Geometry: see drawing. Coordinates: mm, zero at the bounding-box minimum. Give positions to 0.01 mm unless a question says otherwise; leave off trailing zeros. Order: outer loops, then holes, each group sorted by start corner. A loop starts at its lowest first (then second) coordinate and runs counter-clockwise, first axis right, second up. Notation, with made-up numbers: M 3.5,43.25 L 57.5,43.25 A23 ccw 57.5,79.25 Z; hole C 82.5,-27.5 d5. An arc over 180 degrees is marked long. Return JSON: item names as keys, results as strings.
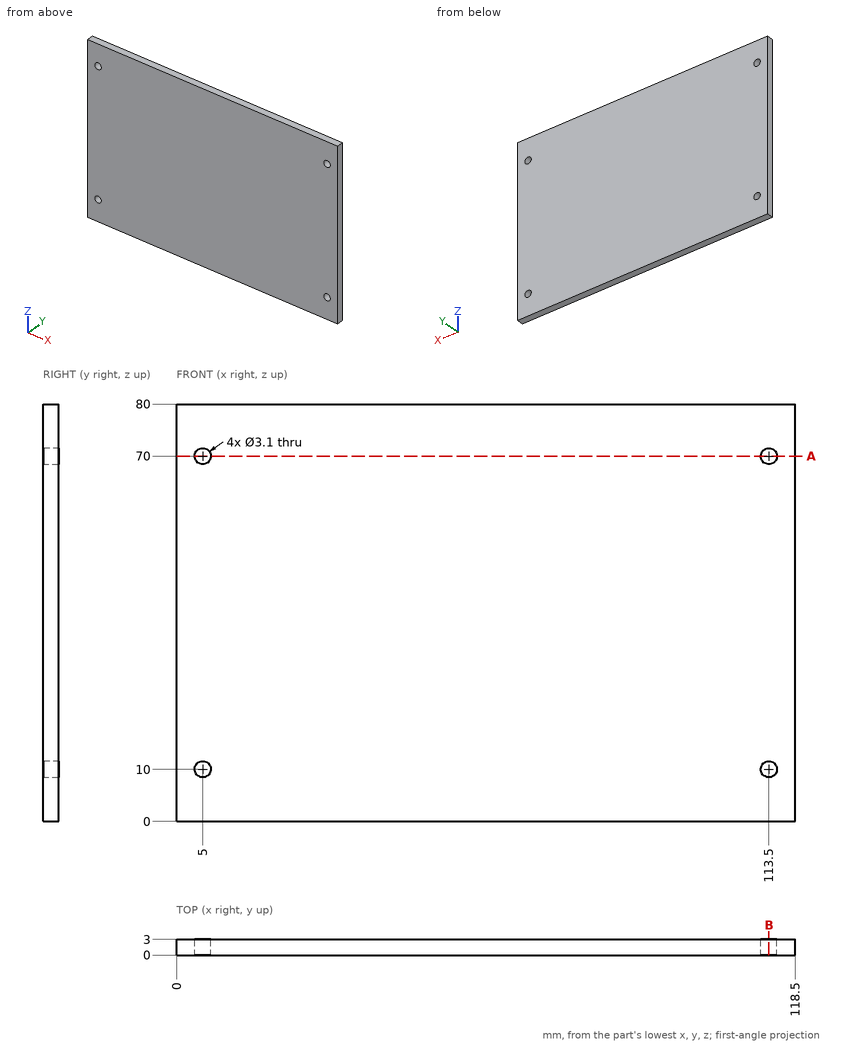
1. First-contact query: pin 1 (2.5 mm diameter, centred on x = 113.5, z = 10, fed in from -Y). Flat tip, straight axial feed; report the tip coordinate or a pass-through.
Evaluation:
{"pin 1": "passes through"}
2. Section query B-B (x = 113.5). Return loops of the section in (y, z), then the cut area to 3 significant figures.
Evaluation:
{"outline": "M 0,0 L 3,0 L 3,8.45 L 0,8.45 Z; M 0,11.55 L 3,11.55 L 3,68.45 L 0,68.45 Z; M 0,71.55 L 3,71.55 L 3,80 L 0,80 Z", "area": "221 mm^2"}
3. Section query A-A (z = 70). Return loops of the section in (x, y), then the cut area to 3 significant figures.
Evaluation:
{"outline": "M 0,0 L 3.45,0 L 3.45,3 L 0,3 Z; M 6.55,0 L 111.95,0 L 111.95,3 L 6.55,3 Z; M 115.05,0 L 118.5,0 L 118.5,3 L 115.05,3 Z", "area": "337 mm^2"}
4. Ray query, probe 1 along X at (y, z) = (2, 10); probe 2 along Z at (x, y) = (113.5, 2.15). Return the intervals inside material, ascending.
Evaluation:
{"probe 1": "x = 0 to 3.45, 6.55 to 111.95, 115.05 to 118.5", "probe 2": "z = 0 to 8.45, 11.55 to 68.45, 71.55 to 80"}
